```python
from build123d import *

# Parameters (mm, degrees)
SKETCH1_R           = 17.5
BOSS_EXTRUDE1_DEPTH = 65
SKETCH2_R           = 35
BOSS_EXTRUDE2_DEPTH = 12.7
SKETCH3_R           = 18
BOSS_EXTRUDE3_DEPTH = 31.6
SKETCH4_W           = 73.126959069
SKETCH4_H           = 81
BOSS_EXTRUDE4_DEPTH = 62.2


with BuildPart() as part:
    # Sketch1 → Boss-Extrude1 (new body)
    with BuildSketch(Plane(origin=(0, 0, 0), x_dir=(0, 0, -1), z_dir=(1, 0, 0))):
        Circle(SKETCH1_R)
    extrude(amount=-BOSS_EXTRUDE1_DEPTH)

    # Sketch2 → Boss-Extrude2 (add)
    with BuildSketch(Plane(origin=(0, 0, 0), x_dir=(0, 0, -1), z_dir=(1, 0, 0))):
        Circle(SKETCH2_R)
    extrude(amount=BOSS_EXTRUDE2_DEPTH)

    # Sketch3 → Boss-Extrude3 (add)
    with BuildSketch(Plane(origin=(12.7, 0, 0), x_dir=(0, 0, -1), z_dir=(1, 0, 0))):
        Circle(SKETCH3_R)
    extrude(amount=BOSS_EXTRUDE3_DEPTH)

    # Sketch4 → Boss-Extrude4 (add)
    with BuildSketch(Plane(origin=(44.3, 0, 0), x_dir=(0, 0, -1), z_dir=(1, 0, 0))):
        with Locations((0.590599522, 3.829138734)):
            Rectangle(SKETCH4_W, SKETCH4_H)
    extrude(amount=BOSS_EXTRUDE4_DEPTH)


solid = part.part
```
Input: part model. Units: mm. Frame: model coordinates. A direction names the side the tool comes from. Coordinates: 2 decimals unless noted, no trailing zeros. Loops run counter-clockwise (first coordinate to the right, second up) from the corner with the lowest first, then second, coordinate; pieces in that order, holes last. Notation, with made-up numbers: M 15,63.25 L 41,63.25 A21 cw 41,90.25 Z; hole C -10,30.5 d8. An arc over 180 degrees is marked long. One line per item, written item: value.
(1) Section C-C (y = 21). Output: boundary loops of the cut face in (x, z).
Filled in:
outline: M 0,-28 L 12.7,-28 L 12.7,28 L 0,28 Z; M 44.3,-37.15 L 106.5,-37.15 L 106.5,35.97 L 44.3,35.97 Z
(2) Section A-A (z = 0). Output: boundary loops of the cut face in (x, y).
Filled in:
outline: M -65,-17.5 L 0,-17.5 L 0,-35 L 12.7,-35 L 12.7,-18 L 44.3,-18 L 44.3,-36.67 L 106.5,-36.67 L 106.5,44.33 L 44.3,44.33 L 44.3,18 L 12.7,18 L 12.7,35 L 0,35 L 0,17.5 L -65,17.5 Z
(3) Reachability of faces 4 (the cylindrical face through (28.279, 17.847, 2.343)), 5 (the flat face through (-65, 0, 0)), 6 (the cylindrical face through (-32.045, -10.648, 13.887)) from +Z, -Z, +X, -X, +Y, -Y: full face, straight path, thin tool, end or side. Return the list, or none.
Filled in:
face 4: none
face 5: +Z, -Z, -X, +Y, -Y
face 6: -X
(4) Pull-direction query (X, two-part tool) for faces 1 (the flat face through (75, 3, 35.973)), 2 (the flat face through (44.3, 22, 0)), 3 (the flat face through (0, 16, 8)); classes: +X half, -X half, draft (parallel to the pull), parting line (faces both ways), or undercut.
Filled in:
face 1: draft
face 2: undercut
face 3: -X half
(5) Section D-D (z = 29). Output: boundary loops of the cut face in (x, y).
Filled in:
outline: M 0,-19.6 L 12.7,-19.6 L 12.7,19.6 L 0,19.6 Z; M 44.3,-36.67 L 106.5,-36.67 L 106.5,44.33 L 44.3,44.33 Z
(6) Section B-B (y = 0). Output: boundary loops of the cut face in (x, z), and give its area (3 significant figures).
Filled in:
outline: M -65,-17.5 L 0,-17.5 L 0,-35 L 12.7,-35 L 12.7,-18 L 44.3,-18 L 44.3,-37.15 L 106.5,-37.15 L 106.5,35.97 L 44.3,35.97 L 44.3,18 L 12.7,18 L 12.7,35 L 0,35 L 0,17.5 L -65,17.5 Z
area: 8,850 mm^2
(7) Pin query (flat end, axial travel): pin 1 (2 mm diameter, centred on y = -4.5, z = -29.5, fed in from -X); pin 2 (1.5 mm diameter, centred on y = 32.5, z = 15.5, fed in from -X). Return the tip coordinate at first contact, or that it passes through.
Filled in:
pin 1: x = 0
pin 2: x = 44.3
(8) Line query: line 1 along X through (y, z) = (22, 26); line 2 along X through (y, z) = (41.5, 0); line 3 along X through (y, z) = (13.5, 11.5). Output: solid intervals per line, ascending. Write a range as from..to.
Filled in:
line 1: 0..12.7, 44.3..106.5
line 2: 44.3..106.5
line 3: 0..106.5
